from build123d import *

# Parameters (mm, degrees)
SKETCH_1_R          = 15
SKETCH_1_R_2        = 1.6
EXTRUDE_1_DEPTH     = 16
SKETCH_2_W          = 40
SKETCH_2_H          = 10
CUT_EXTRUDE_1_DEPTH = 10
FILLET_2_R          = 5


with BuildPart() as part:
    # ｽｹｯﾁ1 → ﾎﾞｽ - 押し出し1 (new body)
    with BuildSketch(Plane.XY):
        with BuildLine():
            Line((20, 25), (-20, 25))
            Line((-20, 25), (-20, -5))
            ThreePointArc((-20, -5), (-14.142135624, -19.142135624), (0, -25))
            ThreePointArc((0, -25), (14.142135624, -19.142135624), (20, -5))
            Line((20, -5), (20, 25))
        make_face()
        with Locations((0, -5)):
            Circle(SKETCH_1_R, mode=Mode.SUBTRACT)
        with Locations((-15, 20)):
            Circle(SKETCH_1_R_2, mode=Mode.SUBTRACT)
        with Locations((15, 20)):
            Circle(SKETCH_1_R_2, mode=Mode.SUBTRACT)
    extrude(amount=EXTRUDE_1_DEPTH)

    # ｽｹｯﾁ2 → ｶｯﾄ - 押し出し1 (cut)
    with BuildSketch(Plane(origin=(0, 25, 0), x_dir=(1, 0, 0), z_dir=(0, 1, 0))):
        with Locations((0, -8)):
            Rectangle(SKETCH_2_W, SKETCH_2_H)
    extrude(amount=-CUT_EXTRUDE_1_DEPTH, mode=Mode.SUBTRACT)

    # ﾌｨﾚｯﾄ2
    fillet_2_edges = [part.edges().sort_by_distance(p)[0] for p in [
        (-20, 25, 14.5),
        (20, 25, 14.5),
        (-20, 25, 1.5),
        (20, 25, 1.5),
    ]]
    fillet(fillet_2_edges, radius=FILLET_2_R)


solid = part.part
The model under review builds one solid part; all positions refer to its coordinate system, in mm. A direction names the side the tool comes from. Round coordinates to 2 decimals unless told otherwise and drop trailing zeros. Loops run counter-clockwise (first coordinate to the right, second up) from the corner with the lowest first, then second, coordinate; pieces in that order, holes last. Notation, with made-up numbers: M 19,71.25 L 69,71.25 A23 cw 69,88.25 Z; hole C 34,39 d10. An arc over 180 degrees is marked long. Answer as a JSON object with one key per item and string values.
Item 1: Tool access review of faces 1 (the face through (0, 20, 13)), 2 (the face through (-18, 24, 2)): name each direction out of +Z, -Z, +X, -X, +Y, -Y from which nothing blocks a thin tool from reaching the whole face with its end or side.
Check sheet entries:
{"face 1": "+X, -X, +Y", "face 2": "+Z, -Z, -X, +Y"}
Item 2: The part is to be moulded in two halves that separate along Z. For faces 3 (the face through (0, 15, 8)), 4 (the face through (0, 11, 0)), 5 (the face through (-16.18, 21.08, 14.48)), say which applies: +Z half, -Z half, draft (parallel to the pull), parting line (faces both ways), or undercut.
Check sheet entries:
{"face 3": "undercut", "face 4": "-Z half", "face 5": "draft"}
Item 3: We need section B-B, the plane y = 1. State the section outline as (x, z) points, and give its area (3 significant figures).
Check sheet entries:
{"outline": "M -20,0 L -13.75,0 L -13.75,16 L -20,16 Z; M 13.75,0 L 20,0 L 20,16 L 13.75,16 Z", "area": "200 mm2"}
Item 4: We need section D-D, the plane y = 6. State the section outline as (x, z) points, and give its area (3 significant figures).
Check sheet entries:
{"outline": "M -20,0 L -10.2,0 L -10.2,16 L -20,16 Z; M 10.2,0 L 20,0 L 20,16 L 10.2,16 Z", "area": "314 mm2"}
Item 5: We need section A-A, the plane x = 12. State the section outline as (y, z) points, and give its area (3 significant figures).
Check sheet entries:
{"outline": "M -21,0 L -14,0 L -14,16 L -21,16 Z; M 4,0 L 25,0 L 25,3 L 15,3 L 15,13 L 25,13 L 25,16 L 4,16 Z", "area": "348 mm2"}
Item 6: We need section C-C, the plane z = 4.25. State the section outline as (x, y) points.
Check sheet entries:
{"outline": "M -20,-5 A20 ccw 20,-5 L 20,15 L -20,15 Z; hole C 0,-5 d30"}
Item 7: For line 1 along X through (y, z) = (20, 1.8); line 2 along Z through (x, y) = (-14.5, 18); line 3 along X through (y, z) = (-12, 14) (1 decimal), list the stretches that pass through material, from the lowest coordinate up.
Check sheet entries:
{"line 1": "-20 to -16.6, -13.4 to 13.4, 16.6 to 20", "line 2": "0 to 3, 13 to 16", "line 3": "-18.7 to -13.3, 13.3 to 18.7"}
Item 8: Clearance check with flat-ended pins moving along their axes: P1, Ø8, axis at x = -4, y = 1.5, coming from the -Z side; P2, Ø1.5, axis at y = -17.5, z = 3.5, coming from the -X side; P3, Ø4, axis at x = 3.5, z = 12.5, coming from the -Y side; P4, Ø3, axis at x = -2.5, z = 9, coming from the +Y side. State where each tip first meets the part, or that it passes through.
Check sheet entries:
{"P1": "through", "P2": "x = -16.18", "P3": "y = -24.94", "P4": "y = 15"}
